```python
from build123d import *

# Parameters (mm, degrees)
SKETCH1_W               = 108.761980125
SKETCH1_H               = 61.936744186
BOSS_EXTRUDE1_DEPTH     = 2
SKETCH2_R               = 1.5
CUT_EXTRUDE1_DEPTH      = 63.943741049
MIRROR2_COPY_1_SKETCH_R = 1.5
MIRROR2_COPY_1_DEPTH    = 63.943741049
SKETCH3_W               = 94.024869854
SKETCH3_H               = 56.555498618
CUT_EXTRUDE2_DEPTH      = 63.943741049
SKETCH6_W               = 101.2762547
SKETCH6_H               = 61.936744186
CUT_EXTRUDE5_DEPTH      = 10
SKETCH8_W               = 0.808555921
SKETCH8_H               = 61.936744186
BOSS_EXTRUDE2_DEPTH     = 4


with BuildPart() as part:
    # Sketch1 → Boss-Extrude1 (new body)
    with BuildSketch(Plane(origin=(0, 0, 0), x_dir=(1, 0, 0), z_dir=(0, 1, 0))):
        with Locations((-0.380990063, 0)):
            Rectangle(SKETCH1_W, SKETCH1_H)
    extrude(amount=BOSS_EXTRUDE1_DEPTH)

    # Sketch2 → Cut-Extrude1 (cut, through all)
    with BuildSketch(Plane(origin=(0, 2, 0), x_dir=(1, 0, 0), z_dir=(0, 1, 0))):
        with Locations(Location((-50.921572875, 27.996572875, 0), (0, 0, 270))):
            Circle(SKETCH2_R)
    cut_extrude1 = extrude(amount=-CUT_EXTRUDE1_DEPTH, mode=Mode.SUBTRACT)

    # Mirror1: Cut-Extrude1 across plane
    add(cut_extrude1.mirror(Plane.XY), mode=Mode.SUBTRACT)

    # Mirror2: Cut-Extrude1 across plane
    add(cut_extrude1.mirror(Plane.ZY.offset(0.380990062)), mode=Mode.SUBTRACT)

    # Mirror2 copy 1 sketch → Mirror2 copy 1 (cut, through all)
    with BuildSketch(Plane(origin=(-0.761980125, 2, 0), x_dir=(-1, 0, 0), z_dir=(0, 1, 0))):
        with Locations(Location((-50.921572875, 27.996572875, 0), (0, 0, 270))):
            Circle(MIRROR2_COPY_1_SKETCH_R)
    extrude(amount=-MIRROR2_COPY_1_DEPTH, mode=Mode.SUBTRACT)

    # Sketch3 → Cut-Extrude2 (cut, through all)
    with BuildSketch(Plane(origin=(0, 2, 0), x_dir=(1, 0, 0), z_dir=(0, 1, 0))):
        Rectangle(SKETCH3_W, SKETCH3_H)
    extrude(amount=-CUT_EXTRUDE2_DEPTH, mode=Mode.SUBTRACT)

    # Sketch6 → Cut-Extrude5 (cut)
    with BuildSketch(Plane(origin=(0, 2, 0), x_dir=(1, 0, 0), z_dir=(0, 1, 0))):
        with Locations((3.36187265, 0)):
            Rectangle(SKETCH6_W, SKETCH6_H)
    extrude(amount=-CUT_EXTRUDE5_DEPTH, mode=Mode.SUBTRACT)

    # Sketch8 → Boss-Extrude2 (add)
    with BuildSketch(Plane(origin=(0, 2, 0), x_dir=(1, 0, 0), z_dir=(0, 1, 0))):
        with Locations((-55.166258086, 0)):
            Rectangle(SKETCH8_W, SKETCH8_H)
    extrude(amount=-BOSS_EXTRUDE2_DEPTH)


solid = part.part
```
The listing builds one solid part. Answer for the finished solid, in the listing's coordinates (mm). A direction names the side the tool comes from. Coordinates: 2 decimals unless noted, no trailing zeros. Write each loop counter-clockwise with the first axis right and the second up, starting at its lowest first coordinate (ties: lowest second). Pieces come first, ordered by that corner, then holes. Notation, with made-up numbers: M -15.75,36.5 L -10.75,36.5 A17 cw -10.75,56.5 Z; hole C 37.25,-3.75 d9. An arc over 180 degrees is marked long. Use a Markdown table: item, result. Add a question column.
1. Section B-B (x = -51.5) is taken. Give the vertices of the cut face in (y, z).
2. Section A-A (z = 21.5) is taken. Give the vertices of the cut face in (x, y), plus the area to 3 significant figures.
3. Given P1, Ø2, axis at x = -52.5, z = -7, coming from the -Y side; P2, Ø0.6, axis at y = -1, z = 9, coming from the +X side, each flat-ended and moving along its own axis, determine where each tip first touches the part or whether it passes through.
4. For a pull along X with two mould halves and no side action, classify faces 1 (the flat face through (-51, 2, 0)), 2 (the cylindrical face through (-49.908, 1.014, -29.102)), 3 (the flat face through (-47.276, 1, 0)) as +X half, -X half, draft (parallel to the pull), parting line (faces both ways), or undercut.
5. Section D-D (x = -48.25) is taken. Give the vertices of the cut face in (y, z), plus the area to 3 significant figures.
6. Which of the six approach directions +Z, -Z, +X, -X, +Y, -Y give full straight-line access (tool end or side, diameter ignored) to faces 4 (the flat face through (-55.571, 0, 0)), 5 (the flat face through (-54.762, -1, 0))?
7. Section C-C (y = -0.75) is taken. Give the vertices of the cut face in (x, z), plus the area to 3 significant figures.
8. Straight lines are drawn through the part: line 1 along Z through (x, y) = (-51, 0.5); line 2 along Y through (x, z) = (-48.5, -14); line 3 along X through (y, z) = (-1.65, 15). For each, find the intervals that lie inside material, in ascending order. Write a range as [from, to].
Data:
| question | item | result |
|---|---|---|
| 1 | outline | M 0,-30.97 L 2,-30.97 L 2,-29.38 L 0,-29.38 Z; M 0,-26.61 L 2,-26.61 L 2,26.61 L 0,26.61 Z; M 0,29.38 L 2,29.38 L 2,30.97 L 0,30.97 Z |
| 2 | outline | M -55.57,-2 L -54.76,-2 L -54.76,0 L -47.28,0 L -47.28,2 L -55.57,2 Z |
| 2 | area | 18.2 mm2 |
| 3 | P1 | stops at y = 0 |
| 3 | P2 | stops at x = -54.76 |
| 4 | face 1 | draft |
| 4 | face 2 | undercut |
| 4 | face 3 | +X half |
| 5 | outline | M 0,-30.97 L 2,-30.97 L 2,30.97 L 0,30.97 Z |
| 5 | area | 124 mm2 |
| 6 | face 4 | +Z, -Z, -X, +Y, -Y |
| 6 | face 5 | +Z, -Z, +X, -Y |
| 7 | outline | M -55.57,-30.97 L -54.76,-30.97 L -54.76,30.97 L -55.57,30.97 Z |
| 7 | area | 50.1 mm2 |
| 8 | line 1 | z = [-30.97, -29.49], [-26.5, 26.5], [29.49, 30.97] |
| 8 | line 2 | y = [0, 2] |
| 8 | line 3 | x = [-55.57, -54.76] |
